The listing builds one solid part. Answer for the finished solid, in the listing's coordinates (mm). A direction names the side the tool comes from. Round coordinates to 2 decimals unless told otherwise and drop trailing zeros. Write each loop counter-clockwise with the first axis right and the second up, starting at its lowest first coordinate (ties: lowest second). Pieces come first, ordered by that corner, then holes. Notation, with made-up numbers: M -16,71 L -7,71 A28 cw -7,110 Z; hole C -17.75,50.5 d3. An arc over 180 degrees is marked long. Write each question's results on one line, items separated by ' | '.
from build123d import *

# Parameters (mm, degrees)
SKETCH1_R                 = 15.4
BOSS_EXTRUDE1_DEPTH       = 20
BOSS_EXTRUDE2_DEPTH       = 20
FILLET4_R                 = 8
CIRPATTERN11_COUNT        = 2
FILLET4_OF_CIRPATTERN11_R = 8
SKETCH4_R                 = 14
CUT_EXTRUDE3_DEPTH        = 18
SKETCH5_R                 = 5
CUT_EXTRUDE4_DEPTH        = 19
CUT_EXTRUDE4_DEPTH_BACK   = 3
CUT_EXTRUDE5_START        = -3
SKETCH7_R                 = 3
CUT_EXTRUDE5_DEPTH        = 22
CIRPATTERN12_COUNT        = 4
CUT_EXTRUDE1_START        = -21
SKETCH2_R                 = 1.5
CUT_EXTRUDE1_DEPTH        = 22
CIRPATTERN10_COUNT        = 2
SKETCH3_R                 = 5.75
CUT_EXTRUDE2_DEPTH        = 2.5
CIRPATTERN3_COUNT         = 2
MIRROR1_COPY_1_SKETCH_R   = 5.75
MIRROR1_COPY_1_DEPTH      = 2.5


with BuildPart() as part:
    # Sketch1 → Boss-Extrude1 (new body)
    with BuildSketch(Plane.XY):
        Circle(SKETCH1_R)
    extrude(amount=BOSS_EXTRUDE1_DEPTH)

    # Sketch6 → Boss-Extrude2 (add)
    with BuildSketch(Plane.XY.offset(20)):
        with BuildLine():
            Line((-23.675, 3), (-15.104966071, 3))
            ThreePointArc((-15.104966071, 3), (-15.4, 0), (-15.104966071, -3))
            Line((-15.104966071, -3), (-23.675, -3))
            ThreePointArc((-23.675, -3), (-26.675, 0), (-23.675, 3))
        make_face()
    boss_extrude2 = extrude(amount=-BOSS_EXTRUDE2_DEPTH)

    # Fillet4
    fillet4_edges = [part.edges().sort_by_distance(p)[0] for p in [
        (-15.104966071, 3, 10),
        (-15.104966071, -3, 10),
    ]]
    fillet(fillet4_edges, radius=FILLET4_R)

    # CirPattern11: Boss-Extrude2 ×2 about axis
    cirpattern11_axis = Axis((0, 0, 0), (0, 0, 1))
    for i in range(1, CIRPATTERN11_COUNT):
        add(boss_extrude2.rotate(cirpattern11_axis, i * 360 / CIRPATTERN11_COUNT))

    # Fillet4 of CirPattern11
    fillet4_of_cirpattern11_edges = [part.edges().sort_by_distance(p)[0] for p in [
        (15.104966071, -3, 10),
        (15.104966071, 3, 10),
    ]]
    fillet(fillet4_of_cirpattern11_edges, radius=FILLET4_OF_CIRPATTERN11_R)

    # Sketch4 → Cut-Extrude3 (cut)
    with BuildSketch(Plane.XY.offset(20)):
        Circle(SKETCH4_R)
    extrude(amount=-CUT_EXTRUDE3_DEPTH, mode=Mode.SUBTRACT)

    # Sketch5 → Cut-Extrude4 (cut, two sides)
    with BuildSketch(Plane.XY.offset(2)) as cut_extrude4_sk:
        Circle(SKETCH5_R)
    extrude(amount=CUT_EXTRUDE4_DEPTH, mode=Mode.SUBTRACT)
    extrude(cut_extrude4_sk.sketch, amount=-CUT_EXTRUDE4_DEPTH_BACK, mode=Mode.SUBTRACT)

    # Sketch7 → Cut-Extrude5 (cut)
    with BuildSketch(Plane.XY.offset(2).offset(CUT_EXTRUDE5_START)):
        with Locations((-8.4, 0)):
            Circle(SKETCH7_R)
    cut_extrude5 = extrude(amount=CUT_EXTRUDE5_DEPTH, mode=Mode.SUBTRACT)

    # CirPattern12: Cut-Extrude5 ×4 about axis
    cirpattern12_axis = Axis((0, 0, 0), (0, 0, 1))
    for i in range(1, CIRPATTERN12_COUNT):
        add(cut_extrude5.rotate(cirpattern12_axis, i * 360 / CIRPATTERN12_COUNT), mode=Mode.SUBTRACT)

    # Sketch2 → Cut-Extrude1 (cut)
    with BuildSketch(Plane.XY.offset(20).offset(CUT_EXTRUDE1_START)):
        with Locations((-23.675, 0)):
            Circle(SKETCH2_R)
    cut_extrude1 = extrude(amount=CUT_EXTRUDE1_DEPTH, mode=Mode.SUBTRACT)

    # CirPattern10: Cut-Extrude1 ×2 about axis
    cirpattern10_axis = Axis((0, 0, 0), (0, 0, 1))
    for i in range(1, CIRPATTERN10_COUNT):
        add(cut_extrude1.rotate(cirpattern10_axis, i * 360 / CIRPATTERN10_COUNT), mode=Mode.SUBTRACT)

    # Sketch3 → Cut-Extrude2 (cut, symmetric)
    with BuildSketch(Plane.XY.offset(5.771567898)):
        with Locations((-23.675, 0)):
            Circle(SKETCH3_R)
    cut_extrude2 = extrude(amount=CUT_EXTRUDE2_DEPTH, both=True, mode=Mode.SUBTRACT)

    # CirPattern3: Cut-Extrude2 ×2 about axis
    cirpattern3_axis = Axis((0, 0, 0), (0, 0, 1))
    for i in range(1, CIRPATTERN3_COUNT):
        add(cut_extrude2.rotate(cirpattern3_axis, i * 360 / CIRPATTERN3_COUNT), mode=Mode.SUBTRACT)

    # Mirror1: Cut-Extrude2 across plane
    add(cut_extrude2.mirror(Plane.XY.offset(10)), mode=Mode.SUBTRACT)

    # Mirror1 copy 1 sketch → Mirror1 copy 1 (cut, symmetric)
    with BuildSketch(Plane(origin=(0, 0, 14.228432102), x_dir=(-1, 0, 0), z_dir=(0, 0, -1))):
        with Locations((-23.675, 0)):
            Circle(MIRROR1_COPY_1_SKETCH_R)
    extrude(amount=MIRROR1_COPY_1_DEPTH, both=True, mode=Mode.SUBTRACT)


solid = part.part
1) Section C-C (y = 8.4) is taken. Determine the outline of the cut face in (x, z), then the cut area to 3 significant figures.
Return value:
outline: M -12.91,0 L -3,0 L -3,2 L -11.2,2 L -11.2,20 L -12.91,20 Z; M 3,0 L 12.91,0 L 12.91,20 L 11.2,20 L 11.2,2 L 3,2 Z | area: 101 mm²
2) Find the intervals of material crossed by line 1 (Y direction, x = 0, z = 16.25); line 2 (Y direction, x = 3.5, z = 2.25); line 3 (X direction, y = 8, z = 12.5), in increasing order.
Return value:
line 1: -15.4 to -14, 14 to 15.4 | line 2: -15 to -13.56, 13.56 to 15 | line 3: -13.16 to -11.49, 11.49 to 13.16
3) The mould has two halves that part along Z. Classify faces 1 (the face through (-4, -14, 20)), 2 (the face through (22, 3, 18)), 3 (the face through (21, 0, 3.272)): +Z half, -Z half, draft (parallel to the pull), parting line (faces both ways), or undercut.
Return value:
face 1: +Z half | face 2: draft | face 3: undercut
4) Section B-B (z = 9.5) is taken. Determine the outline of the cut face in (x, y) (3 decimals).
Return value:
outline: M -23.675,-3 L -20.653,-3 A8 cw -13.592,-7.239 A15.4 ccw 13.592,-7.239 A8 cw 20.653,-3 L 23.675,-3 A3 ccw 23.675,3 L 20.653,3 A8 cw 13.592,7.239 A15.4 ccw -13.592,7.239 A8 cw -20.653,3 L -23.675,3 A3 ccw Z; hole C -23.675,0 d3; hole C 0,0 d28; hole C 23.675,0 d3
5) Each of these flat-tipped pins is pushed along its axis until it touches: pin 1 (3.5 mm diameter, centred on x = -22.5, z = 10, fed in from -Y); pin 2 (5 mm diameter, centred on x = -8.4, y = 0, fed in from -Z); pin 3 (8 mm diameter, centred on y = -8, z = 15, fed in from -X); pin 4 (4 mm diameter, centred on x = -18.5, z = 15.5, fed in from -Y). Where does it stop, or does it pass through?
Return value:
pin 1: y = -3 | pin 2: through | pin 3: x = -16.78 | pin 4: y = -4.16
6) Section A-A (x = 0) is taken. Determine the outline of the cut face in (y, z), then the cut area to 3 significant figures.
Return value:
outline: M -15.4,0 L -11.4,0 L -11.4,2 L -14,2 L -14,20 L -15.4,20 Z; M -5.4,0 L -5,0 L -5,2 L -5.4,2 Z; M 5,0 L 5.4,0 L 5.4,2 L 5,2 Z; M 11.4,0 L 15.4,0 L 15.4,20 L 14,20 L 14,2 L 11.4,2 Z | area: 68.0 mm²
7) A tool of negligible diameter and unlimited length cuts with its end or side. For faces 4 (the face through (26.674, 0.066, 1.659)), 5 (the face through (-22, -3, 10)), 6 (the face through (22, -3, 18)), 7 (the face through (-11.4, 0.1, 1)), 8 (the face through (-22, 3, 18)), from which of +Z, -Z, +X, -X, +Y, -Y can it reach the whole face along a straight path? Write none if from no direction.
Return value:
face 4: +Z, -Z, +X | face 5: +Z, -Z, -X, -Y | face 6: +Z, -Z, +X, -Y | face 7: +Z, -Z | face 8: +Z, -Z, -X, +Y
